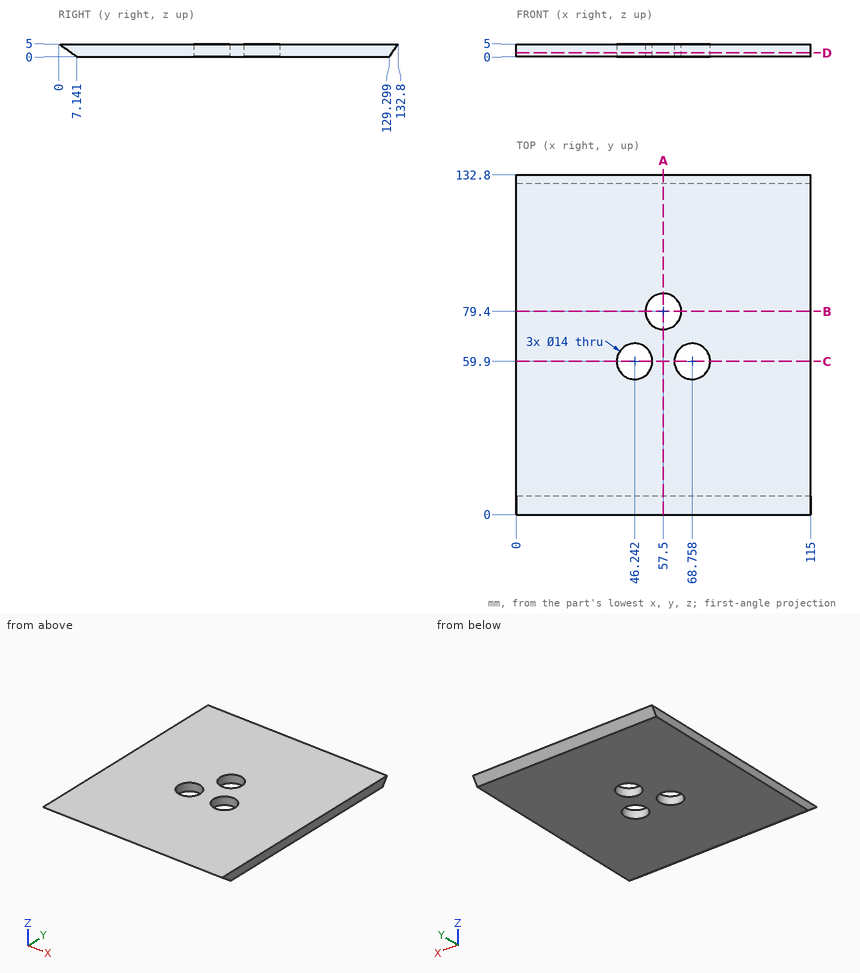
Design review of the part shown in the three views and the two pictorial views. Dimensions are in mm from the part's minimum x, y and z. Give positions to 0.01 mm unless a question says otherwise; leave off trailing zeros. Write each loop counter-clockwise with the first axis right and the second up, starting at its lowest first coordinate (ties: lowest second). Pieces come first, ordered by that corner, then holes.
(1) Add section B-B (y = 79.4). Give the boundary of the cut face in (x, z), and give its area (3 significant figures).
Checked values:
outline: (0, 0) - (50.5, 0) - (50.5, 5) - (0, 5) - close; (64.5, 0) - (115, 0) - (115, 5) - (64.5, 5) - close
area: 505 mm2
(2) Clearance check with flat-ended pins moving along their axes: pin 1 Ø8.5 at (x, y) = (46.24, 59.9) entering from -Z; pin 2 Ø1.5 at (x, z) = (57, 2.5) entering from +Y (1 decimal); pin 3 Ø2 at (x, z) = (18, 1.5) entering from +Y. State where each tip first meets the part, or that it passes through.
Checked values:
pin 1: passes through
pin 2: stops at y = 131.6
pin 3: stops at y = 131.05
(3) Add section D-D (z = 1.5). Give the boundary of the cut face in (x, y), and give its area (3 significant figures).
Checked values:
outline: (0, 5) - (115, 5) - (115, 130.35) - (0, 130.35) - close; hole circle Ø14 at (46.24, 59.9); hole circle Ø14 at (57.5, 79.4); hole circle Ø14 at (68.76, 59.9)
area: 14,000 mm2
(4) Wall thickness on line 1 along Y through (x, z) = (57.5, 3.5); line 2 along Y through (x, z) = (66.5, 3.3) (1 decimal); line 3 along Y through (x, z) = (106, 1.5): over which ranges is each line inside the solid? List them lowest first.
Checked values:
line 1: y = 2.14 to 72.4, 86.4 to 131.75
line 2: y = 2.4 to 53.3, 66.5 to 131.6
line 3: y = 5 to 130.35
(5) Add section C-C (y = 59.9). Give the boundary of the cut face in (x, z), and give its area (3 significant figures).
Checked values:
outline: (0, 0) - (39.24, 0) - (39.24, 5) - (0, 5) - close; (53.24, 0) - (61.76, 0) - (61.76, 5) - (53.24, 5) - close; (75.76, 0) - (115, 0) - (115, 5) - (75.76, 5) - close
area: 435 mm2
(6) Add section A-A (x = 57.5). Give the boundary of the cut face in (y, z).
Checked values:
outline: (0, 5) - (7.14, 0) - (72.4, 0) - (72.4, 5) - close; (86.4, 0) - (129.3, 0) - (132.8, 5) - (86.4, 5) - close
